Here's how the part is built. I have some questions about the finished solid (model axes, mm). A direction names the side the tool comes from. Coordinates: 2 decimals unless noted, no trailing zeros. Order: outer loops, then holes, each group sorted by start corner. A loop starts at its lowest first (then second) coordinate and runs counter-clockwise, first axis right, second up. Notation, with made-up numbers: (6.5, -26) -> (20.5, -26) arc R11 ccw to (20.5, -6) -> close; hole circle Ø2 at (-23.5, 68.25). An arc over 180 degrees is marked (long way). One line per item, written item: value. Start each with the question number.
```python
from build123d import *

# Parameters (mm, degrees)
BOSS_EXTRUDE1_DEPTH = 5
SKETCH2_R           = 2.25
CUT_EXTRUDE1_DEPTH  = 28.910571474
CHAMFER1_SIZE       = 2
SKETCH4_W           = 10
SKETCH4_H           = 8
CUT_EXTRUDE3_DEPTH  = 15
SKETCH3_R           = 1.65
CUT_EXTRUDE2_DEPTH  = 35.799425283


with BuildPart() as part:
    # Sketch1 → Boss-Extrude1 (new, symmetric)
    with BuildSketch(Plane.XY):
        Polygon((-23, -15), (23, -15), (23, -10), (8, -10), (8, 5), (-8, 5), (-8, -10), (-23, -10), align=None)
    extrude(amount=BOSS_EXTRUDE1_DEPTH, both=True)

    # Sketch2 → Cut-Extrude1 (cut, through all)
    with BuildSketch(Plane(origin=(0, -10, 0), x_dir=(1, 0, 0), z_dir=(0, 1, 0))):
        with Locations(Location((-15.5, 0, 0), (0, 0, 180))):
            Circle(SKETCH2_R)
        with Locations(Location((15.5, 0, 0), (0, 0, 180))):
            Circle(SKETCH2_R)
    extrude(amount=-CUT_EXTRUDE1_DEPTH, mode=Mode.SUBTRACT)

    # Chamfer1
    chamfer1_edges = [part.edges().sort_by_distance(p)[0] for p in [
        (-13.25, -10, 0),
        (17.75, -10, 0),
    ]]
    chamfer(chamfer1_edges, length=CHAMFER1_SIZE)

    # Sketch4 → Cut-Extrude3 (cut)
    with BuildSketch(Plane(origin=(0, 5, 0), x_dir=(1, 0, 0), z_dir=(0, 1, 0))):
        with Locations((0, 1)):
            Rectangle(SKETCH4_W, SKETCH4_H)
    extrude(amount=-CUT_EXTRUDE3_DEPTH, mode=Mode.SUBTRACT)

    # Sketch3 → Cut-Extrude2 (cut, through all)
    with BuildSketch(Plane(origin=(8, 0, 0), x_dir=(0, 0, -1), z_dir=(1, 0, 0))):
        with Locations(Location((1, 0, 0), (0, 0, 90))):
            Circle(SKETCH3_R)
    extrude(amount=-CUT_EXTRUDE2_DEPTH, mode=Mode.SUBTRACT)


solid = part.part
```
Q1. Imagine slicing it at B-B (y = 0). Write out the boundary of the cut face in (x, z).
Q2. For P1, Ø5, axis at x = -13.5, z = -2.5, coming from the +Y side; P2, Ø3, axis at y = -3.5, z = 2, coming from the -X side; P3, Ø3, axis at y = -4.5, z = 2, coming from the +X side; P4, Ø2.5, axis at x = -15.5, z = 0, coming from the +Y side, each with a flat end and sliding along its axis, tell me the tip position at first contact or that it passes through.
Q3. I need wall thicknesses on line 1 (X direction, y = -4, z = -2.75); line 2 (Z direction, x = -15.5, y = -13.8); line 3 (Z direction, x = 6, y = 0). Which ranges of each line are inside material? Lowest first, please.
Q4. For faces 1 (the face through (0, -2, 3)), 2 (the face through (-15.4, -10, -4.4)), 3 (the face through (8, -3, 0)), which set-ups out of +Z, -Z, +X, -X, +Y, -Y let a thin tool reach every point of the face, with its end or its side?
Q5. If we mould it in two halves opening along Y, with no side actions, what happens to faces 4 (the face through (0, -15, 0)), 5 (the face through (0.1, 5, 3.4)), 6 (the face through (6.5, -0.4, -2.6)), 7 (the face through (-5, -2, -1))? For each: +Y half, -Y half, draft (parallel to the pull), parting line (faces both ways), or undercut.
Q6. Imagine slicing it at D-D (z = 0). Count the separate pieces of the cut face and the enclosed holes in it, plus the area to 3 significant figures.
Q7. Imagine slicing it at C-C (y = -6.5). Write out the boundary of the cut face in (x, z), plus the area to 3 significant figures.
Q8. Imagine slicing it at A-A (x = 15.5). Write out the boundary of the cut face in (y, z), plus the area to 3 significant figures.
Completed:
1. outline: (-8, -5) -> (-5, -5) -> (-5, -2.65) -> (-8, -2.65) -> close; (-8, 0.65) -> (-5, 0.65) -> (-5, 3) -> (5, 3) -> (5, 0.65) -> (8, 0.65) -> (8, 5) -> (-8, 5) -> close; (5, -5) -> (8, -5) -> (8, -2.65) -> (5, -2.65) -> close
2. P1: stops at y = -10
2. P2: stops at x = -8
2. P3: stops at x = 8
2. P4: passes through
3. line 1: x = -8 to -5, 5 to 8
3. line 2: z = -5 to -2.25, 2.25 to 5
3. line 3: z = -5 to -2.65, 0.65 to 5
4. face 1: -Z, +Y
4. face 2: +Z, -Z, -X, +Y
4. face 3: +Z, -Z, +X, +Y
5. face 4: -Y half
5. face 5: +Y half
5. face 6: undercut
5. face 7: draft
6. separate pieces: 5
6. enclosed holes: 0
6. area: 251 mm2
7. outline: (-8, -5) -> (-5, -5) -> (-5, 3) -> (5, 3) -> (5, -5) -> (8, -5) -> (8, 5) -> (-8, 5) -> close
7. area: 80.0 mm2
8. outline: (-15, -5) -> (-10, -5) -> (-10, -4.25) -> (-12, -2.25) -> (-15, -2.25) -> close; (-15, 2.25) -> (-12, 2.25) -> (-10, 4.25) -> (-10, 5) -> (-15, 5) -> close
8. area: 23.5 mm2
